Read the model definition and answer for the solid it produces. Units are mm, in the model's axes. Face numbers are marked on the shaded views. A direction names the side the tool comes from. Round coordinates to 2 decimals unless told otherwise and drop trailing zeros. Write each loop counter-clockwise with the first axis right and the second up, starting at its lowest first coordinate (ties: lowest second). Pieces come first, ordered by that corner, then holes. Notation, with made-up numbers: (40, 14) -> (45, 14) arc R30 ccw to (45, 48) -> close; hole circle Ø9 at (32, -2.5). An arc over 180 degrees is marked (long way). Return JSON: item names as keys, results as strings.
from build123d import *

# Parameters (mm, degrees)
F0_W      = 50.8
F0_H      = 50.8
F1_DEPTH  = 1005.84
F3_DEPTH  = 50.8
F4_W      = 1371.6
F4_H      = 50.8
F5_DEPTH  = 50.8
F11_DEPTH = 955.04


# Not quite as in the source:
# - a feature of the source that left no trace in its solid (it failed there, or was rolled back) is left out


with BuildPart() as f1:
    # F0 (on Front) → F1 (new body)
    with BuildSketch(Plane.XZ):
        with Locations((-1295.4, 683.9833942235)):
            Rectangle(F0_W, F0_H)
        with Locations((25.4, 683.9833942235)):
            Rectangle(F0_W, F0_H)
        Polygon((-1270, 0), (0, 0), (0, 658.5833942235), (0, 709.3833942235), (-1270, 709.3833942235), (-1270, 658.5833942235), align=None)
    extrude(amount=-F1_DEPTH)

    # F2 (on face) → F3 (join)
    with BuildSketch(Plane(origin=(0, 1005.84, 0), x_dir=(-1, 0, 0), z_dir=(0, 1, 0))):
        Polygon((1320.8, 709.3833942235), (914.4, 709.3833942235), (914.4, 658.5833942235), (1270, 658.5833942235), (1320.8, 658.5833942235), align=None)
        Polygon((-50.8, 709.3833942235), (-50.8, 658.5833942235), (0, 658.5833942235), (355.6, 658.5833942235), (355.6, 709.3833942235), align=None)
    extrude(amount=F3_DEPTH)

    # F4 (on face) → F5 (join)
    with BuildSketch(Plane.XZ):
        with Locations((-635, 683.9833942235)):
            Rectangle(F4_W, F4_H)
    extrude(amount=F5_DEPTH)

    # F10 (on face) → F11 (cut)
    with BuildSketch(Plane(origin=(0, 1005.84, 0), x_dir=(-1, 0, 0), z_dir=(0, 1, 0))):
        Polygon((355.6, 709.3833942235), (355.6, 658.5833942235), (355.6, 113.7688308954), (914.4, 113.7688308954), (914.4, 658.5833942235), (914.4, 709.3833942235), align=None)
        Polygon((355.6, 113.7688308954), (355.6, 658.5833942235), (0, 658.5833942235), (0, 0), (1270, 0), (1270, 658.5833942235), (914.4, 658.5833942235), (914.4, 113.7688308954), align=None)
    extrude(amount=-F11_DEPTH, mode=Mode.SUBTRACT)


solid = f1.part
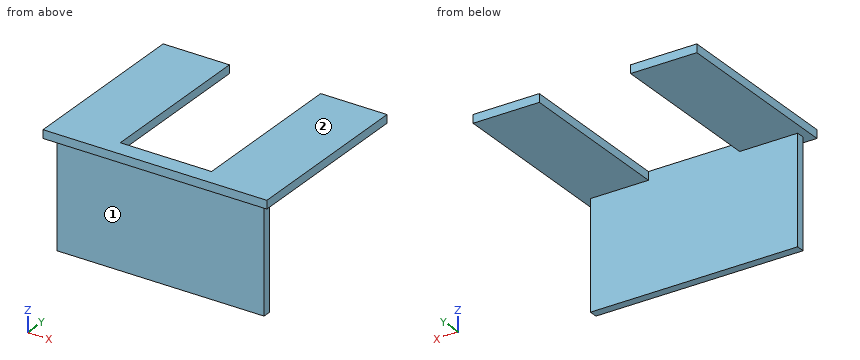
Item 1: Section A-A (y = 706.5) is taken. Give the vertices of the cut face in (x, z).
Worked answers:
{"outline": "(-1320.8, 658.58) -> (-914.4, 658.58) -> (-914.4, 709.38) -> (-1320.8, 709.38) -> close; (-355.6, 658.58) -> (50.8, 658.58) -> (50.8, 709.38) -> (-355.6, 709.38) -> close"}
Item 2: Section C-C (z = 340.5) is taken. Give the vertices of the cut face in (x, y), then the cut area to 3 significant figures.
Worked answers:
{"outline": "(-1270, 0) -> (0, 0) -> (0, 50.8) -> (-1270, 50.8) -> close", "area": "64,500 mm2"}
Item 3: Section D-D (x = -872.5) is taken. Give the vertices of the cut face in (y, z), then the cut area to 3 significant figures.
Worked answers:
{"outline": "(-50.8, 658.58) -> (0, 658.58) -> (0, 0) -> (50.8, 0) -> (50.8, 709.38) -> (-50.8, 709.38) -> close", "area": "38,600 mm2"}
Item 4: A tool of negligible diameter and unlimited length cuts with its end or side. For the marked faces 1 and 2, from which of +Z, -Z, +X, -X, +Y, -Y can it reach the whole face along a straight path? Write none if from no direction.
Worked answers:
{"face 1": "-Z, +X, -X, -Y", "face 2": "+Z, +X, -X, +Y, -Y"}
Item 5: Flat-ended cylindrical pins translate along their axes: pin 1 (6 mm diameter, centred on x = -1124, y = 129.5, fed in from -Z); pin 2 (10 mm diameter, centred on x = -817, z = 395, fed in from +Y). Find the tip coordinate at first contact, or state that the pin passes through.
Worked answers:
{"pin 1": "stops at z = 658.58", "pin 2": "stops at y = 50.8"}
Item 6: Section B-B (x = -70) is taken. Give the vertices of the cut face in (y, z), then the cut area to 3 significant figures.
Worked answers:
{"outline": "(-50.8, 658.58) -> (0, 658.58) -> (0, 0) -> (50.8, 0) -> (50.8, 658.58) -> (1056.64, 658.58) -> (1056.64, 709.38) -> (-50.8, 709.38) -> close", "area": "89,700 mm2"}
Item 7: Straight lines are drawn through the part: L1, parallel to Y at x = -1121.5, z = 208; L2, parallel to Z at x = -1251, y = 783. For each, find the intervals that lie inside material, in ascending order. Write a range as [from, to].
Worked answers:
{"L1": "y = [0, 50.8]", "L2": "z = [658.58, 709.38]"}
